from build123d import *

# Parameters (mm, degrees)
BOSS_EXTRUDE1_DEPTH              = 2.54
FILLET1_R                        = 1.27
F_97_0_0059_DIAMETER_HOLE2_D     = 0.508
F_97_0_0059_DIAMETER_HOLE2_DEPTH = 25.4
F_97_0_0059_DIAMETER_HOLE2_TIP   = 0.152618597


with BuildPart() as part:
    # Sketch1 → Boss-Extrude1 (new body)
    with BuildSketch(Plane(origin=(0, 0, 0), x_dir=(1, 0, 0), z_dir=(0, 1, 0))):
        Polygon((0, 0), (6.35, 0), (6.35, 5.08), (-3.302, 5.08), (-3.302, 0), align=None)
    extrude(amount=BOSS_EXTRUDE1_DEPTH)

    # Fillet1
    fillet1_edges = [part.edges().sort_by_distance(p)[0] for p in [
        (-3.302, 0, -2.54),
        (-3.302, 2.54, -2.54),
    ]]
    fillet(fillet1_edges, radius=FILLET1_R - 0.0001)  # a hair under: the kernel refuses the full size

    # #97 (0.0059) Diameter Hole2
    with Locations(Plane.XY):
        with Locations((6.35, 1.27)):
            Hole(F_97_0_0059_DIAMETER_HOLE2_D / 2, depth=F_97_0_0059_DIAMETER_HOLE2_DEPTH)
            with Locations((0, 0, -(F_97_0_0059_DIAMETER_HOLE2_DEPTH + F_97_0_0059_DIAMETER_HOLE2_TIP / 2))):  # 118° drill point
                Cone(0, F_97_0_0059_DIAMETER_HOLE2_D / 2, F_97_0_0059_DIAMETER_HOLE2_TIP, mode=Mode.SUBTRACT)


solid = part.part
Verification items for the finished model (mm, model axes). Coordinates: 2 decimals unless noted, no trailing zeros. Order: outer loops, then holes, each group sorted by start corner. A loop starts at its lowest first (then second) coordinate and runs counter-clockwise, first axis right, second up. Notation, with made-up numbers: M 87,49.25 L 121,49.25 A37 ccw 121,87.25 Z; hole C 37.25,-31 d5. An arc over 180 degrees is marked long. One line per item, written item: value. Start each with the question number.
Item 1: Sectioned sample at C-C on y = 2. Record the cut outline in (x, z).
Item 2: Thickness scan on probe 1 along X at (y, z) = (1.25, -1.3); probe 2 along X at (y, z) = (2, -2.6). Record the ranges inside material, lowest first.
Item 3: Mould release check, pull along Z, two halves, no side actions. Record for faces 1 (the flat face through (1, 1, 0)), 2 (the flat face through (2, 1, -5.08)), 3 (the cylindrical face through (-2.94, 0.38, -2.5)): pulls with the +Z half, pulls with the -Z half, needs draft (parallel to the pull), parting line crosses it, or undercut.
Item 4: Sectioned sample at B-B on y = 0.3. Record the cut outline in (x, z).
Calculated:
1. outline: M -3.07,-5.08 L 6.35,-5.08 L 6.35,0 L -3.07,0 Z
2. probe 1: -3.3 to 6.1
2. probe 2: -3.07 to 6.35
3. face 1: pulls with the +Z half
3. face 2: pulls with the -Z half
3. face 3: needs draft
4. outline: M -2.85,-5.08 L 6.35,-5.08 L 6.35,0 L -2.85,0 Z
